Verification items for the finished model (mm, model axes). A direction names the side the tool comes from. Coordinates: 2 decimals unless noted, no trailing zeros. Order: outer loops, then holes, each group sorted by start corner. A loop starts at its lowest first (then second) coordinate and runs counter-clockwise, first axis right, second up. Notation, with made-up numbers: M 55,64 L 104,64 A18 cw 104,78 Z; hole C 18.5,19.25 d2. An arc over 180 degrees is marked long. Answer as a JSON object with one key per item and string values. Group by question number.
(1) Gauge pin test, flat ends, axial feed: pin 1 Ø1 at (y, z) = (26.5, 76) entering from +X; pin 2 Ø1 at (x, y) = (1.5, 24.5) entering from -Z. Record the tip position at first contact, or that the pin passes through.
(2) Mould release check, pull along Z, two halves, no side actions. Record for faces 1 (the face through (-107.5, 25.8, 98.6)), 2 (the face through (-41, 26, 200)), 3 (the face through (-41, 26.802, 10)), 4 (the face through (-41, 26, 0)): released by +Z, released by -Z, zero draft, split by the parting line, or undercut.
(3) Access from +Z, -Z, +X, -X, +Y, -Y to the whole of each face (thin tool, end or side, straight path). Record for faces 5 (the face through (-42, 28.302, 99)), 6 (the face through (-45.8, 27.6, 12.2)).
(4) Cross-section at B-B (y = 25.9). Enter the section's corners in (x, z), plus the area to 3 significant figures.
(5) Cross-section at A-A (z = 10). Enter the section's corners in (x, y).
(6) Material ranges on line 1 (X direction, y = 27.55, z = 10); line 2 (X direction, y = 27.15, z = 10); line 3 (Z direction, x = -39, y = 28.05), recorded low to high.
from build123d import *

# Parameters (mm, degrees)
BOSS_EXTRUDE1_DEPTH = 200
SKETCH2_R           = 4.828226571
CUT_EXTRUDE1_DEPTH  = 1.5


with BuildPart() as part:
    # Sketch1 → Boss-Extrude1 (new body)
    with BuildSketch(Plane.XY):
        Polygon((-106.5, 28.302180685), (23.5, 28.302180685), (25.5, 23.302180685), (-108.5, 23.302180685), align=None)
    extrude(amount=BOSS_EXTRUDE1_DEPTH)

    # Sketch2 → Cut-Extrude1 (cut)
    with BuildSketch(Plane(origin=(0, 28.302180685, 0), x_dir=(1, 0, 0), z_dir=(0, 1, 0))):
        with Locations(Location((-41.5, -10, 0), (0, 0, 270))):
            Circle(SKETCH2_R)
    extrude(amount=-CUT_EXTRUDE1_DEPTH, mode=Mode.SUBTRACT)


solid = part.part
Taken from the geometry:
{
 "1": {"pin 1": "stops at x = 24.42", "pin 2": "stops at z = 0"},
 "2": {"face 1": "zero draft", "face 2": "released by +Z", "face 3": "undercut", "face 4": "released by -Z"},
 "3": {"face 5": "+Z, -Z, +X, -X, +Y", "face 6": "+Y"},
 "4": {"outline": "M -107.46,0 L 24.46,0 L 24.46,200 L -107.46,200 Z", "area": "26,400 mm²"},
 "5": {"outline": "M -108.5,23.3 L 25.5,23.3 L 23.5,28.3 L -36.67,28.3 L -36.67,26.8 L -46.33,26.8 L -46.33,28.3 L -106.5,28.3 Z"},
 "6": {"line 1": "x = -106.8 to -46.33, -36.67 to 23.8", "line 2": "x = -106.96 to -46.33, -36.67 to 23.96", "line 3": "z = 0 to 5.87, 14.13 to 200"}
}
